Design review of the part built by this model. Coordinates are the model's own, in mm. Face numbers are marked on the shaded views. Give positions to 0.01 mm unless a question says otherwise; leave off trailing zeros. Answer as a JSON object with one key per item and string values.
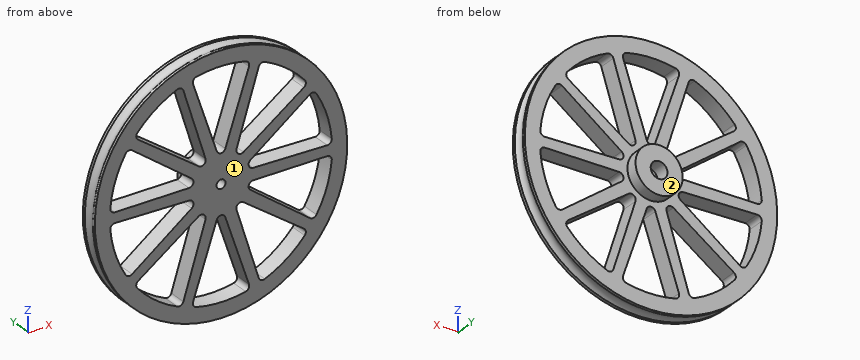
from build123d import *

# Parameters (mm, degrees)
BOSS_EXTRUDE1_DEPTH = 3
CIRPATTERN1_COUNT   = 10
BOSS_EXTRUDE2_DEPTH = 3
CIRPATTERN3_COUNT   = 10


with BuildPart() as part:
    # Sketch2 → Revolve1 (revolve)
    with BuildSketch(Plane.XY, mode=Mode.PRIVATE) as revolve1_sk:
        Polygon((2.841205436, -5), (7.841205436, -5), (7.841205436, 5), (2.794, 5), (2.794, 0), (1.5, 0), (1.5, -5), align=None)
        with BuildLine():
            Line((42, -4), (42, -5))
            Line((42, -5), (37, -5))
            Line((37, -5), (37, 1))
            Line((37, 1), (42, 1))
            Line((42, 1), (42, 0))
            add(Edge.make_bspline(
                [(42, 0), (40.4125, -2), (42, -4)],
                knots=[0, 0, 0, 1, 1, 1], degree=2))
        make_face()
    revolve(revolve1_sk.sketch.rotate(Axis((0, 0, 0), (0, 1, 0)), 90), axis=Axis((0, 0, 0), (0, 1, 0)))

    # Sketch3 → Boss-Extrude1 (add, symmetric)
    with BuildSketch(Plane(origin=(0, -2, 0), x_dir=(1, 0, 0), z_dir=(0, 1, 0))):
        with BuildLine():
            Line((7.581853512, 2), (36.961862454, 1.679501106))
            ThreePointArc((36.961862454, 1.679501106), (37, 0), (36.961862454, -1.679501106))
            Line((36.961862454, -1.679501106), (7.581853512, -2))
            ThreePointArc((7.581853512, -2), (7.841205436, 0), (7.581853512, 2))
        make_face()
    boss_extrude1 = extrude(amount=BOSS_EXTRUDE1_DEPTH, both=True)

    # CirPattern1: Boss-Extrude1 ×10 about axis
    cirpattern1_axis = Axis((0, 0, 0), (0, 1, 0))
    for i in range(1, CIRPATTERN1_COUNT):
        add(boss_extrude1.rotate(cirpattern1_axis, i * 360 / CIRPATTERN1_COUNT))

    # Sketch4 → Boss-Extrude2 (add, symmetric)
    with BuildSketch(Plane(origin=(0, -2, 0), x_dir=(1, 0, 0), z_dir=(0, 1, 0))):
        with BuildLine():
            Line((4.958277836, -6.074535668), (7.461905948, -7.852127938))
            ThreePointArc((7.461905948, -7.852127938), (5.711839894, -7.861673162), (5.161961694, -9.523135251))
            Line((5.161961694, -9.523135251), (4.245034617, -6.5927372))
            ThreePointArc((4.245034617, -6.5927372), (4.608944915, -6.343668454), (4.958277836, -6.074535668))
        make_face()
        with BuildLine():
            Line((13.019144113, -34.633825757), (12.534602349, -33.085283591))
            ThreePointArc((12.534602349, -33.085283591), (13.338668476, -33.999791988), (14.556277797, -34.016389825))
            ThreePointArc((14.556277797, -34.016389825), (13.791166744, -34.333711128), (13.019144113, -34.633825757))
        make_face()
        with BuildLine():
            Line((27.592569409, -22.145030136), (28.915588887, -23.084382585))
            ThreePointArc((28.915588887, -23.084382585), (28.391594801, -23.725879218), (27.853371989, -24.355485395))
            ThreePointArc((27.853371989, -24.355485395), (28.213848481, -23.192341103), (27.592569409, -22.145030136))
        make_face()
    boss_extrude2 = extrude(amount=BOSS_EXTRUDE2_DEPTH, both=True)

    # CirPattern3: Boss-Extrude2 ×10 about axis
    cirpattern3_axis = Axis((0, 0, 0), (0, 1, 0))
    for i in range(1, CIRPATTERN3_COUNT):
        add(boss_extrude2.rotate(cirpattern3_axis, i * 360 / CIRPATTERN3_COUNT))


solid = part.part
(1) Insertion check: pin 1 (3 mm diameter, centred on x = 31.5, y = -2.5, fed in from -Z); pin 2 (1.5 mm diameter, centred on x = -10, y = 2.5, fed in from +Z); pin 3 (1 mm diameter, centred on x = -28, y = -0.5, fed in from +Z); pin 4 (2 mm diameter, centred on x = -19, y = 0, fed in from +Z). Each pin has a flat end and moves straight along its axis. Give the tip position at first contact, or say it passes through.
Checked values:
{"pin 1": "stops at z = -28.5", "pin 2": "passes through", "pin 3": "stops at z = 31.47", "pin 4": "stops at z = 37.95"}
(2) We need section A-A (x = -34). Count the separate pieces of the cut face and the enclosed holes in it, plus the area to 3 significant figures.
Checked values:
{"separate pieces": "3", "enclosed holes": "0", "area": "134 mm^2"}
(3) To check wall thickness, follow L1, parallel to Z at x = 2, y = 1.25; L2, parallel to X at y = -4.25, z = 32.5; L3, parallel to Z at x = 15, y = -0.25. State the ranges of each line that lie inside material, in increasing order. Write a range as from..to.
Checked values:
{"L1": "z = -7.58..-1.95, 1.95..7.58", "L2": "x = -26.6..-17.68, -12.35..-8.76, 8.76..12.35, 17.68..26.6", "L3": "z = -39.03..-33.82, -13.2..-8.56, -1.92..1.92, 8.56..13.2, 33.82..39.03"}
(4) Draft analysis for pull direction Y (two halves, no side actions). For the marked faces 1 and 2, state which applies: +Y half, -Y half, draft (parallel to the pull), parting line (faces both ways), or undercut.
Checked values:
{"face 1": "-Y half", "face 2": "+Y half"}
